```python
from build123d import *

# Parameters (mm, degrees)
SKETCH1_W           = 68.6
SKETCH1_H           = 53.3
BOSS_EXTRUDE1_DEPTH = 1
SKETCH2_R           = 1.3
BOSS_EXTRUDE2_DEPTH = 8


with BuildPart() as part:
    # Sketch1 → Boss-Extrude1 (new body)
    with BuildSketch(Plane.XY):
        with Locations((34.3, 26.65)):
            Rectangle(SKETCH1_W, SKETCH1_H)
    extrude(amount=BOSS_EXTRUDE1_DEPTH)

    # Sketch2 → Boss-Extrude2 (add)
    with BuildSketch(Plane.XY.offset(1)):
        with Locations(Location((14, 2.5, 0), (0, 0, 180))):
            Circle(SKETCH2_R)
        with Locations(Location((15.3, 50.8, 0), (0, 0, 180))):
            Circle(SKETCH2_R)
        with Locations(Location((66.1, 7.6, 0), (0, 0, 180))):
            Circle(SKETCH2_R)
        with Locations(Location((66.1, 35.5, 0), (0, 0, 180))):
            Circle(SKETCH2_R)
    extrude(amount=BOSS_EXTRUDE2_DEPTH)


solid = part.part
```
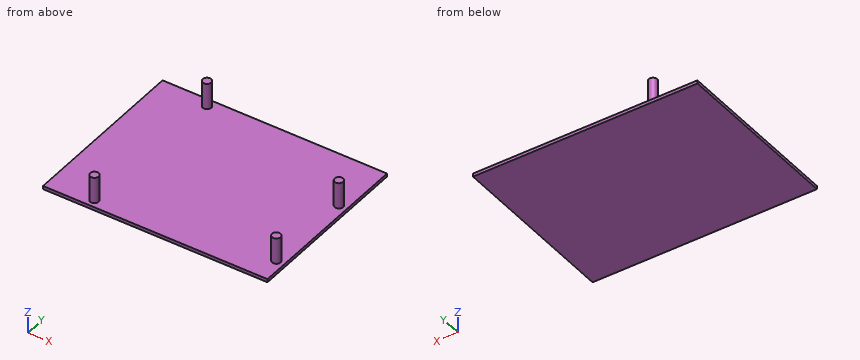
Work out the finished part from the listing and answer in its coordinate system (mm). Coordinates: 2 decimals unless noted, no trailing zeros. Loops run counter-clockwise (first coordinate to the right, second up) from the corner with the lowest first, then second, coordinate; pieces in that order, holes last. Notation, with made-up numbers: M 64.25,-9 L 119.25,-9 A13 cw 119.25,-5 Z; hole C -39.75,69 d6. An arc over 180 degrees is marked long. Use CSV: the item, a comma, the result in double quotes. Start each with the question number.
(1) Find section B-B, the plane y = 7.6. Give the vertices of the cut face in (x, z), then the cut area to 3 significant figures.
(2) Find section D-D, the plane y = 20.5. Give the vertices of the cut face in (x, z), then the cut area to 3 significant figures.
(3) Given pin 1 Ø8 at (x, y) = (16, 37) entering from -Z; pin 2 Ø4 at (y, z) = (28.5, 4) entering from +X; pin 3 Ø16 at (x, y) = (26, 31) entering from +Z, each flat-ended and moving along its own axis, determine where each tip first touches the part or whether it passes through.
(4) Find section A-A, the plane x = 66.1. Give the vertices of the cut face in (y, z), then the cut area to 3 significant figures.
(5) Find section C-C, the plane z = 3.5. Give the vertices of the cut face in (x, y).
(6) Consider line 1 (Z direction, x = 30, y = 44.5); line 2 (X direction, y = 7, z = 2); line 3 (X direction, y = 3, z = 7.5). Determine where each line is inside the solid, lowest interval first.
Recorded:
1,outline,"M 0,0 L 68.6,0 L 68.6,1 L 67.4,1 L 67.4,9 L 64.8,9 L 64.8,1 L 0,1 Z"
1,area,"89.4 mm^2"
2,outline,"M 0,0 L 68.6,0 L 68.6,1 L 0,1 Z"
2,area,"68.6 mm^2"
3,pin 1,"stops at z = 0"
3,pin 2,"passes through"
3,pin 3,"stops at z = 1"
4,outline,"M 0,0 L 53.3,0 L 53.3,1 L 36.8,1 L 36.8,9 L 34.2,9 L 34.2,1 L 8.9,1 L 8.9,9 L 6.3,9 L 6.3,1 L 0,1 Z"
4,area,"94.9 mm^2"
5,outline,"C 14,2.5 d2.6; C 15.3,50.8 d2.6; C 66.1,7.6 d2.6; C 66.1,35.5 d2.6"
6,line 1,"z = 0 to 1"
6,line 2,"x = 64.95 to 67.25"
6,line 3,"x = 12.8 to 15.2"
